from build123d import *

# Parameters (mm, degrees)
CROQUIS1_R              = 3
SALIENTE_EXTRUIR1_DEPTH = 5
REDONDEO3_R             = 4


with BuildPart() as part:
    # Croquis1 → Saliente-Extruir1 (new, symmetric)
    with BuildSketch(Plane(origin=(0, 0, 0), x_dir=(-1, 0, 0), z_dir=(0, 1, 0))):
        with BuildLine():
            Line((0, -7.5), (260, -7.5))
            ThreePointArc((260, -7.5), (267.5, 0), (260, 7.5))
            Line((260, 7.5), (0, 7.5))
            ThreePointArc((0, 7.5), (-7.5, 0), (0, -7.5))
        make_face()
        with Locations(Location((0, 0, 0), (0, 0, 90))):
            Circle(CROQUIS1_R, mode=Mode.SUBTRACT)
        with Locations(Location((260, 0, 0), (0, 0, 90))):
            Circle(CROQUIS1_R, mode=Mode.SUBTRACT)
    extrude(amount=SALIENTE_EXTRUIR1_DEPTH, both=True)

    # Redondeo3
    redondeo3_edges = [part.edges().sort_by_distance(p)[0] for p in [
        (7.5, 5, 0),
        (-130, 5, -7.5),
        (-267.5, 5, 0),
        (-130, -5, -7.5),
        (7.5, -5, 0),
        (-130, -5, 7.5),
        (-267.5, -5, 0),
        (-130, 5, 7.5),
    ]]
    fillet(redondeo3_edges, radius=REDONDEO3_R)


solid = part.part
For this review, take the finished solid that the model builds, in its own axes (mm). Coordinates: 2 decimals unless noted, no trailing zeros. Loops run counter-clockwise (first coordinate to the right, second up) from the corner with the lowest first, then second, coordinate; pieces in that order, holes last. Notation, with made-up numbers: (15.5, -12.5) - (32.5, -12.5) arc R24 ccw to (32.5, 7.5) - close; hole circle Ø11 at (36.25, 89.5). An arc over 180 degrees is marked (long way). Return JSON: item names as keys, results as strings.
Item 1: Mouldability with a two-part tool opening along Z and no side actions: class faces 1 (the flat face through (-128, -5, 0)), 2 (the cylindrical face through (-257, 0, 0)), 3 (the cylindrical face through (-267.5, 0.01, -0.16)) as pulls with the +Z half, pulls with the -Z half, needs draft (parallel to the pull), parting line crosses it, or undercut.
Determined:
{"face 1": "needs draft", "face 2": "undercut", "face 3": "parting line crosses it"}
Item 2: Take a section at B-B (x = -150.5). Give the boundary of the cut face in (y, z).
Determined:
{"outline": "(-5, -3.5) arc R4 ccw to (-1, -7.5) - (1, -7.5) arc R4 ccw to (5, -3.5) - (5, 3.5) arc R4 ccw to (1, 7.5) - (-1, 7.5) arc R4 ccw to (-5, 3.5) - close"}
Item 3: Take a section at A-A (z = 0). State how many separate pieces and enclosed holes the cut face has, then the cut area to 3 significant figures.
Determined:
{"separate pieces": "3", "enclosed holes": "0", "area": "2,620 mm2"}
Item 4: Insertion check: pin 1 (3.5 mm diameter, centred on x = 0, z = 0, fed in from -Y); pin 2 (3 mm diameter, centred on y = 2, z = 1.5, fed in from +X); pin 3 (1 mm diameter, centred on y = 1, z = 1.5, fed in from +X); pin 4 (5 mm diameter, centred on y = -3, z = 3.5, fed in from +X). Each pin has a flat end and moves straight along its axis. Give the tip position at first contact, or say it passes through.
Determined:
{"pin 1": "passes through", "pin 2": "stops at x = 7.49", "pin 3": "stops at x = 7.43", "pin 4": "stops at x = 7.32"}
Item 5: For line 1 (X direction, y = 0, z = 0); line 2 (X direction, y = -3, z = -1.5); line 3 (Z direction, x = -260, y = 0.25), list the stretches that pass through material, from the lowest coordinate up.
Determined:
{"line 1": "x = -267.5 to -263, -257 to -3, 3 to 7.5", "line 2": "x = -266.8 to -262.6, -257.4 to -2.6, 2.6 to 6.8", "line 3": "z = -7.5 to -3, 3 to 7.5"}
